Drawing for the job (mm, zero at the part's lowest x, y, z). A direction names the side the tool comes from. Coordinates: 2 decimals unless noted, no trailing zeros. Loops run counter-clockwise (first coordinate to the right, second up) from the corner with the lowest first, then second, coordinate; pieces in that order, holes last. Notation, with made-up numbers: (61, 19.5) -> (77, 19.5) arc R21 ccw to (77, 37.5) -> close; hole circle Ø1 at (-29.75, 15.5). An arc over 180 degrees is marked (long way). Write item = value, one per line. Start each with the question number.
(1) Drill centre lines: line 1 (X direction, y = 20.5, z = 17.5); line 2 (Y direction, x = 23, z = 18); line 3 (X direction, y = 12, z = 5.5). Where is each one in solid material? Low to high. Write a range as from..to.
(2) Band-saw the part on B-B (z = 20). Write the cut outline in (x, y), and give its area (3 significant figures).
(3) Band-saw the part on A-A (y = 20). Write the cut outline in (x, z), and give its area (3 significant figures).
(4) Band-saw the part on C-C (x = 14). Write the cut outline in (y, z).
(5) Tool access for the marked faces 1, 2, 3 and 4: list every direction of +Z, -Z, +X, -X, +Y, -Y with a clear straight run to the whole face (end or side of a thin tool).
(6) Flat gauge pins, fed straight in: P1, Ø5.5, axis at y = 13, z = 13, coming from the +X side; P2, Ø2, axis at y = 35.5, z = 11.5, coming from the +X side; P3, Ø8, axis at x = 35.5, z = 22.5, coming from the -Y side. Where does each tip first touch, or does it go through?
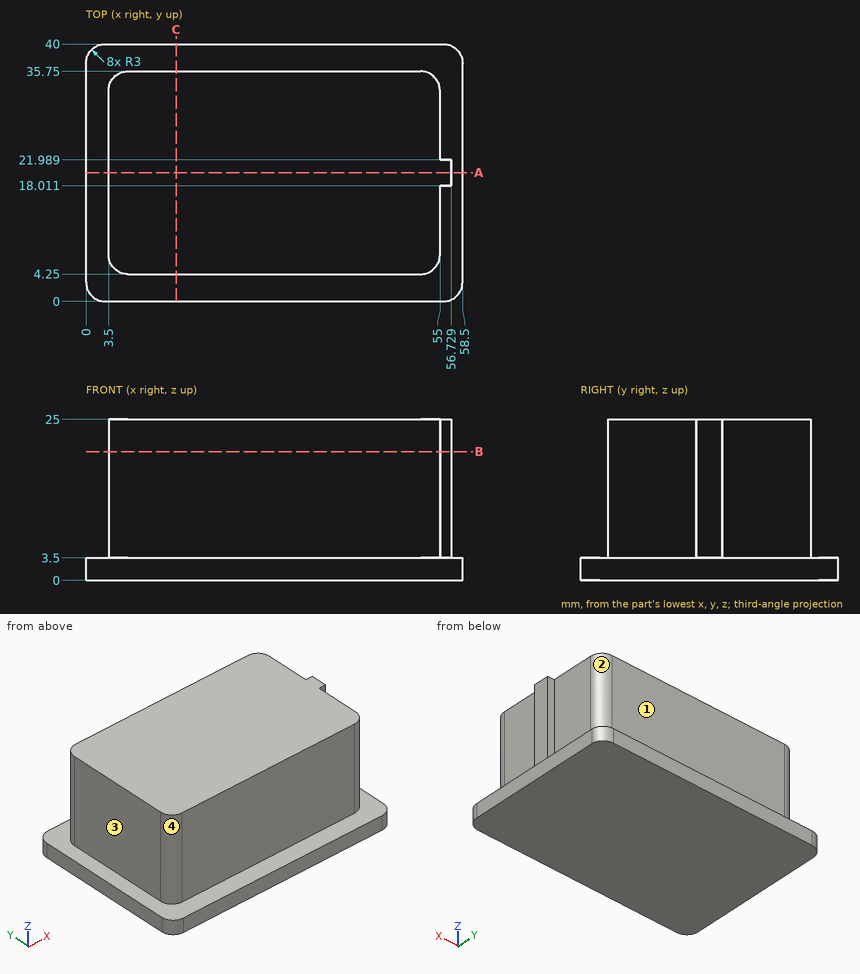
Findings below:
q1.line_1 = 3.5..56.73
q1.line_2 = 4.25..35.75
q1.line_3 = 3.5..55
q2.outline = (3.5, 7.25) arc R3 ccw to (6.5, 4.25) -> (52, 4.25) arc R3 ccw to (55, 7.25) -> (55, 18.01) -> (56.73, 18.01) -> (56.73, 21.99) -> (55, 21.99) -> (55, 32.75) arc R3 ccw to (52, 35.75) -> (6.5, 35.75) arc R3 ccw to (3.5, 32.75) -> close
q2.area = 1,620 mm²
q3.outline = (0, 0) -> (58.5, 0) -> (58.5, 3.5) -> (56.73, 3.5) -> (56.73, 25) -> (3.5, 25) -> (3.5, 3.5) -> (0, 3.5) -> close
q3.area = 1,350 mm²
q4.outline = (0, 0) -> (40, 0) -> (40, 3.5) -> (35.75, 3.5) -> (35.75, 25) -> (4.25, 25) -> (4.25, 3.5) -> (0, 3.5) -> close
q5.face_1 = +Z, +X, -X, +Y
q5.face_2 = +Z, +X, +Y
q5.face_3 = +Z, -X, +Y, -Y
q5.face_4 = +Z, -X, -Y
q6.P1 = 55
q6.P2 = 54.44
q6.P3 = 4.25
